```python
from build123d import *

# Parameters (mm, degrees)
CUT_EXTRUDE1_DEPTH = 3
CHAMFER1_SIZE      = 0.6


with BuildPart() as part:
    # Sketch1 → Revolve1 (revolve)
    with BuildSketch(Plane.XY):
        Polygon((0, 3), (16, 3), (16, 0), (-6, 0), (-6, 5), (0, 5), align=None)
    revolve(axis=Axis((-6, 0, 0), (1, 0, 0)))

    # Sketch2 → Cut-Revolve1 (revolve, cut)
    with BuildSketch(Plane.XY):
        Polygon((-1.497848452, 0), (-3, 2.5), (-6, 2.5), (-6, 0), align=None)
    revolve(axis=Axis((-6, 0, 0), (1, 0, 0)), mode=Mode.SUBTRACT)

    # Sketch3 → Cut-Extrude1 (cut)
    with BuildSketch(Plane.ZY.offset(6)):
        Polygon((2.5, 1.443375673), (0, 2.886751346), (-2.5, 1.443375673), (-2.5, -1.443375673), (0, -2.886751346), (2.5, -1.443375673), align=None)
    extrude(amount=-CUT_EXTRUDE1_DEPTH, mode=Mode.SUBTRACT)

    # Chamfer1
    chamfer1_edges = [part.edges().sort_by_distance(p)[0] for p in [
        (-6, -5, 0),
    ]]
    chamfer(chamfer1_edges, length=CHAMFER1_SIZE)


solid = part.part
```
Verification items for the finished model (mm, model axes). A direction names the side the tool comes from. Coordinates: 2 decimals unless noted, no trailing zeros. Write each loop counter-clockwise with the first axis right and the second up, starting at its lowest first coordinate (ties: lowest second). Pieces come first, ordered by that corner, then holes. Notation, with made-up numbers: M -28,15 L -8,15 A20 cw -8,47 Z; hole C 14,49.5 d6. An arc over 180 degrees is marked long. Answer as a JSON object with one key per item and string values. Group by question number.
(1) Tool access check on faces 4 (the face through (-4.521, 2.155, 1.267)), 5 (the face through (-6, -2, -2)), 6 (the face through (8, -3, 0)). Record the directions out of +Z, -Z, +X, -X, +Y, -Y that give a thin tool (end or side, any length) a straight path to the whole face; none if there is none.
(2) Gauge pin test, flat ends, axial feed: pin 1 (2 mm diameter, centred on x = -1.5, y = -2.5, fed in from +Z); pin 2 (6 mm diameter, centred on x = 9.5, z = 2.5, fed in from -Y). Record the tip position at first contact, or that the pin passes through.
(3) Cross-section at A-A, the plane x = 6. Record the cut outline in (y, z).
(4) Release check for a two-part mould opening along Y. For faces 1 (the face through (-5, 0, -2.5)), 2 (the face through (0, 3.3, 0.1)), 3 (the face through (-2.66, -1.08, -4.88)) record: +Y half, -Y half, draft (parallel to the pull), parting line (faces both ways), or undercut.
(5) Material ranges on line 1 (X direction, y = 3, z = 0.5); line 2 (X direction, y = 1.5, z = 1.75); line 3 (Z direction, x = -3.75, y = 1), recorded low to high.
Reply:
{
 "1": {"face 4": "-X", "face 5": "+Z, -Z, -X, +Y, -Y", "face 6": "+X"},
 "2": {"pin 1": "z = 4.77", "pin 2": "y = -3"},
 "3": {"outline": "C 0,0 d6"},
 "4": {"face 1": "undercut", "face 2": "draft", "face 3": "parting line"},
 "5": {"line 1": "-6 to 0", "line 2": "-2.88 to 16", "line 3": "-4.9 to -2.5, 2.5 to 4.9"}
}
